Geometry check sheet. Reference: the model listing, model coordinates, mm. A direction names the side the tool comes from. Round coordinates to 2 decimals unless told otherwise and drop trailing zeros. Write each loop counter-clockwise with the first axis right and the second up, starting at its lowest first coordinate (ties: lowest second). Pieces come first, ordered by that corner, then holes. Notation, with made-up numbers: (12.5, 40) - (30.5, 40) arc R31 cw to (30.5, 69) - close; hole circle Ø1 at (61.25, -21). An arc over 180 degrees is marked (long way). Return JSON: item names as keys, results as strings.
```python
from build123d import *

# Parameters (mm, degrees)
SKETCH_1_W             = 81.681408993
SKETCH_1_H             = 10
EXTRUDE_1_DEPTH        = 30
EXTRUDE_2_DEPTH        = 30
PATTERN_LINEAR_1_COUNT = 26
PATTERN_LINEAR_1_PITCH = 3.141592654
SKETCH_3_W             = 87.309380436
SKETCH_3_H             = 21.857368967
CUT_EXTRUDE_1_DEPTH    = 20
SKETCH_4_R             = 1.65
CUT_EXTRUDE_4_DEPTH    = 83.8966379


with BuildPart() as part:
    # 草图1 → 拉伸1 (new body)
    with BuildSketch(Plane.XY):
        with Locations((40.840704497, -5)):
            Rectangle(SKETCH_1_W, SKETCH_1_H)
    extrude(amount=EXTRUDE_1_DEPTH)

    # 草图2 → 拉伸2 (add)
    with BuildSketch(Plane.XY.offset(30)):
        Polygon((0, 0), (0.818933027, 2.25), (1.661788885, 2.25), (2.480721912, 0), align=None)
    extrude_2 = extrude(amount=-EXTRUDE_2_DEPTH)

    # 阵列(线性)1: 拉伸2 ×26
    with Locations(*[(i * PATTERN_LINEAR_1_PITCH, 0, 0) for i in range(1, PATTERN_LINEAR_1_COUNT)]):
        add(extrude_2)

    # 草图3 → 切除-拉伸1 (cut)
    with BuildSketch(Plane(origin=(0, 0, 0), x_dir=(-1, 0, 0), z_dir=(0, 0, -1))):
        with Locations((-41.261038515, -3.604772773)):
            Rectangle(SKETCH_3_W, SKETCH_3_H)
    extrude(amount=-CUT_EXTRUDE_1_DEPTH, mode=Mode.SUBTRACT)

    # 草图4 → 切除-拉伸4 (cut, through all)
    with BuildSketch(Plane(origin=(0, 0, 20), x_dir=(-1, 0, 0), z_dir=(0, 0, -1))):
        with Locations((-4.906524017, -3.6)):
            Circle(SKETCH_4_R)
    extrude(amount=-CUT_EXTRUDE_4_DEPTH, mode=Mode.SUBTRACT)


solid = part.part
```
(1) Material ranges on line 1 along X through (y, z) = (-3.75, 24); line 2 along X through (y, z) = (-4.75, 26.75), recorded low to high. Write a range as [from, to].
Response values:
{"line 1": "x = [0, 3.26], [6.55, 81.68]", "line 2": "x = [0, 3.72], [6.09, 81.68]"}
(2) Section check B-B, the plane y = 1.5. Give the number of separate pieces and of enclosed holes in the cut face, plus the area to 3 significant figures.
Response values:
{"separate pieces": "26", "enclosed holes": "0", "area": "361 mm^2"}
(3) Gauge pin test, flat end, axial feed: pin 1 (0.5 mm diameter, centred on x = 6, z = 27, fed in from +Y). Record the tip position at first contact, or that the pin passes through.
Response values:
{"pin 1": "stops at y = 0"}
(4) Access from +Z, -Z, +X, -X, +Y, -Y to the whole of each face (thin tool, end or side, straight path). Record for faces 4 (the face through (0.4, 1.1, 25.1)), 5 (the face through (78.944, 1.109, 25.07)).
Response values:
{"face 4": "+Z, -Z, -X, +Y", "face 5": "+Z, -Z, +Y"}
(5) Section check A-A, the plane y = -3.6. Enter the section's corners in (x, z), plus the area to 3 significant figures.
Response values:
{"outline": "(0, 20) - (3.26, 20) - (3.26, 30) - (0, 30) - close; (6.56, 20) - (81.68, 20) - (81.68, 30) - (6.56, 30) - close", "area": "784 mm^2"}
(6) Release check for a two-part mould opening along Y. For faces 1 (the face through (3.38, -4.23, 24.93)), 2 (the face through (41, -4, 30)), 3 (the face through (41.244, 1.109, 25.07)) record: pulls with the +Y half, pulls with the -Y half, needs draft (parallel to the pull), parting line crosses it, or undercut.
Response values:
{"face 1": "undercut", "face 2": "needs draft", "face 3": "pulls with the +Y half"}
